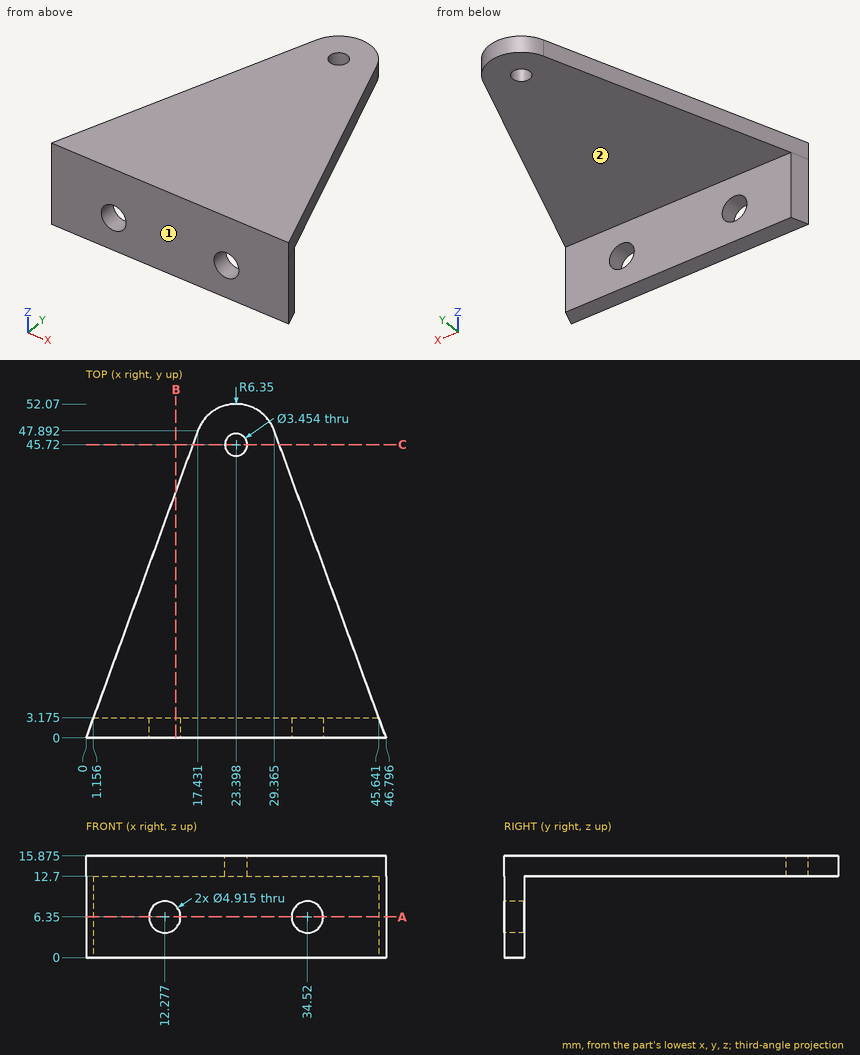
Check sheet for the drawn part. Datum: minimum x, y, z corner. Units: mm. A direction names the side the tool comes from. Round coordinates to 2 decimals unless told otherwise and drop trailing zeros. Write each loop counter-clockwise with the first axis right and the second up, starting at its lowest first coordinate (ties: lowest second). Pieces come first, ordered by that corner, then holes. Notation, with made-up numbers: (-40, -24) -> (-24, -24) arc R18 cw to (-24, -9) -> close; hole circle Ø8 at (13, 86). An arc over 180 degrees is marked (long way). Write each question's results on one line, items separated by ' | '. Start each with the question number.
1. Cross-section at C-C (y = 45.72). Enter the section's corners in (x, z) (1 decimal).
2. Cross-section at B-B (x = 14). Enter the section's corners in (y, z) (1 decimal), then the cut area to 3 significant figures.
3. Material ranges on probe 1 along Y at (x, z) = (29.5, 6) (1 decimal); probe 2 along Z at (x, y) = (41.5, 4.5) (1 decimal); probe 3 along Y at (x, z) = (24, 14.75), recorded low to high. Write a range as from..to.
4. Depth check by flat-ended pin: P1, Ø5.5, axis at x = 34.52, z = 6.35, coming from the +Y side (1 decimal); P2, Ø22, axis at x = 24.5, y = 36, coming from the -Z side. Enter the tip coordinate at first touch or a pass-through.
5. Cross-section at A-A (z = 6.35). Enter the section's corners in (x, y) (1 decimal).
6. Set-up check for the marked faces 1 and 2: record each of +Z, -Z, +X, -X, +Y, -Y from which the full face is reachable in a straight line by a thin tool's end or side.
Solutions:
1) outline: (16.6, 12.7) -> (21.7, 12.7) -> (21.7, 15.9) -> (16.6, 15.9) -> close; (25.1, 12.7) -> (30.2, 12.7) -> (30.2, 15.9) -> (25.1, 15.9) -> close
2) outline: (0, 0) -> (3.2, 0) -> (3.2, 4.6) -> (0, 4.6) -> close; (0, 8.1) -> (3.2, 8.1) -> (3.2, 12.7) -> (38.5, 12.7) -> (38.5, 15.9) -> (0, 15.9) -> close | area: 151 mm2
3) probe 1: y = 0..3.2 | probe 2: z = 12.7..15.9 | probe 3: y = 0..44.1, 47.34..52.04
4) P1: stops at y = 3.2 | P2: stops at z = 12.7
5) outline: (0, 0) -> (9.8, 0) -> (9.8, 3.2) -> (1.2, 3.2) -> close; (14.7, 0) -> (32.1, 0) -> (32.1, 3.2) -> (14.7, 3.2) -> close; (37, 0) -> (46.8, 0) -> (45.6, 3.2) -> (37, 3.2) -> close
6) face 1: +Z, -Z, +X, -X, -Y | face 2: -Z, +X, -X, +Y
